Autodesk Inventor part; units mm, degrees
ref_plane "YZ Plane" through (0, 0, 0) normal (1, 0, 0) x (0, 1, 0)
ref_plane "XZ Plane" through (0, 0, 0) normal (0, 1, 0) x (-1, 0, 0)
ref_plane "XY Plane" through (0, 0, 0) normal (0, 0, 1) x (1, 0, 0)
sketch "Sketch1" plane through (0, 0, 0) normal (0, 1, 0) x (-1, 0, 0)
  line L0 (15.5575, -22.86) -> (15.5575, 27.94)
  line L1 (15.5575, 27.94) -> (-15.5575, 27.94)
  line L2 (-15.5575, 27.94) -> (-15.5575, -22.86)
  line L3 (-15.5575, -27.94) -> (15.5575, 27.94) construction
  line L4 (15.5575, -27.94) -> (-15.5575, 27.94) construction
  line L5 (20.6375, -27.94) -> (20.955, -27.94)
  line L6 (20.955, -27.94) -> (20.955, -78.74)
  line L7 (8.255, -91.44) -> (-8.255, -91.44)
  line L8 (-20.955, -78.74) -> (-20.955, -27.94)
  line L9 (-20.955, -27.94) -> (-20.6375, -27.94)
  arc A0 (15.5575, -22.86) -> (20.6375, -27.94) centre (20.6375, -22.86) ccw
  arc A1 (-20.6375, -27.94) -> (-15.5575, -22.86) centre (-20.6375, -22.86) ccw
  circle A2 centre (0, 7.3025) radius 9.525
  arc A3 (8.255, -91.44) -> (20.955, -78.74) centre (8.255, -78.74) ccw
  arc A4 (-20.955, -78.74) -> (-8.255, -91.44) centre (-8.255, -78.74) ccw
  circle A5 centre (0, -66.04) radius 7.366
  line L10 (0, 46.0525) -> (0, -103.086)
  circle A6 centre (7.62, 21.59) radius 2.3813
  circle A7 centre (-7.62, 21.59) radius 2.3813
  circle A8 centre (12.5412, -34.29) radius 2.3813
  circle A9 centre (-12.5412, -34.29) radius 2.3813
  point P0 (0, 0)
  point P1 (20.955, -91.44)
  point P2 (-20.955, -91.44)
  point P3 (0, 0)
  dimension "d0" = 5.08
  dimension "d1" = 31.115
  dimension "d2" = 41.91
  dimension "d3" = 63.5
  dimension "d4" = 119.38
  dimension "d5" = 19.05
  dimension "d6" = 20.6375
  dimension "d7" = 12.7
  dimension "d27" = 25.4
  dimension "d28" = 14.732
  dimension "d29" = 4.7625
  dimension "d30" = 15.24
  dimension "d31" = 6.35
  dimension "d32" = 25.0825
  dimension "d33" = 4.7625
  dimension "d34" = 57.15
extrude "Extrusion1" add sketch "Sketch1" along normal blind 12.7 contours A0 L5 L6 A3 L7 L10 A5 A2 L1 L0 | L10 A2 A5 L7 A4 L8 L9 A1 L2 L1
sketch "Sketch4" plane through (0, 0, 0) normal (0, -1, 0) x (1, 0, 0)
  circle A0 centre (0, -66.04) radius 7.366
  circle A1 centre (0, -66.04) radius 19.05
  point P0 (0, 0)
  dimension "d38" = 38.1
extrude "Extrusion3" cut sketch "Sketch4" against normal blind 2.54
chamfer "Chamfer1" distance 2.9464 angle 41 2 edges at (10.0013, 0, 21.59) (-5.2387, 0, 21.59) measured on face at (-0.3827, 0, -15.9577)
chamfer "Chamfer2" distance 2.9464 angle 41 2 edges at (-10.16, 12.7, -34.29) (14.9225, 12.7, -34.29) measured on face at (-0.3827, 12.7, -15.9577)
equation "\"d33\" = d29"
properties part number "Fixture_Airpot_Support"
Could you check a few things on this model? Use its own coordinates, in mm. A direction names the side the tool comes from. Round coordinates to 2 decimals unless told otherwise and drop trailing zeros. Write each loop counter-clockwise with the first axis right and the second up, starting at its lowest first coordinate (ties: lowest second). Pieces come first, ordered by that corner, then holes. Notation, with made-up numbers: (32.5, 57) - (52.5, 57) arc R31 ccw to (52.5, 91) - close; hole circle Ø10 at (30.25, 25). An arc over 180 degrees is marked (long way). Put each result on its own line as item: value. Start each with the question number.
(1) I need wall thicknesses on probe 1 along Z at (x, y) = (0, 0.75); probe 2 along Z at (x, y) = (6, 6.25); probe 3 along Z at (x, y) = (-3.5, 4). Which ranges of each line are inside material? Lowest first, please.
(2) Will these pins go through, and if not, where does the flat tip stop? pin 1 (4 mm diameter, centred on x = 13, y = 4, fed in from -Z); pin 2 (4 mm diameter, centred on y = 3.5, z = -4, fed in from +X); pin 3 (3 mm diameter, centred on y = 5.5, z = -12, fed in from -X).
(3) I want a section at B-B, the plane x = 0. Please give me the cut outline in (y, z).
(4) I want a section at C-C, the plane z = 21.59. Please give me the cut outline in (x, y), plus the area to 3 significant figures.
(5) Thinking about a two-plate mould opening in Z: for faces 4 (the cylindrical face through (-7.026, 7.549, -68.253)), 5 (the flat face through (-20.955, 6, -53)), 6 (the flat face through (0, 6, -91.44)), which applies, released by +Z, released by -Z, zero draft, split by the parting line, or undercut?
(6) I want a section at D-D, the plane y = 5.75. Give the number of separate pieces and of enclosed holes in the cut face, plus the area to 3 significant figures.
(7) For faces 1 (the flat face through (8, 2.54, -66)), 2 (the cylindrical face through (-17.333, 6.261, -87.621)), 3 (the flat face through (-15.558, 6, 2)), which set-ups out of +Z, -Z, +X, -X, +Y, -Y let a thin tool reach every point of the face, with its end or its side?
(8) I want a section at A-A, the plane z = -66.04. Please give me the cut outline in (x, y) (3 decimals).
Here are the results:
1. probe 1: z = -91.44 to -85.09, -46.99 to -2.22, 16.83 to 27.94
1. probe 2: z = -91.44 to -70.31, -61.77 to -0.1, 14.7 to 19.84, 23.34 to 27.94
1. probe 3: z = -91.44 to -72.52, -59.56 to -1.56, 16.16 to 27.94
2. pin 1: stops at z = -91.14
2. pin 2: stops at x = 15.56
2. pin 3: stops at x = -15.56
3. outline: (0, -91.44) - (12.7, -91.44) - (12.7, -73.41) - (2.54, -73.41) - (2.54, -85.09) - (0, -85.09) - close; (0, -46.99) - (2.54, -46.99) - (2.54, -58.67) - (12.7, -58.67) - (12.7, -2.22) - (0, -2.22) - close; (0, 16.83) - (12.7, 16.83) - (12.7, 27.94) - (0, 27.94) - close
4. outline: (-15.56, 0) - (-12.95, 0) - (-10, 2.56) - (-10, 12.7) - (-15.56, 12.7) - close; (-5.24, 2.56) - (-2.29, 0) - (2.29, 0) - (5.24, 2.56) - (5.24, 12.7) - (-5.24, 12.7) - close; (10, 2.56) - (12.95, 0) - (15.56, 0) - (15.56, 12.7) - (10, 12.7) - close
4. area: 259 mm^2
5. face 4: undercut
5. face 5: zero draft
5. face 6: released by -Z
6. separate pieces: 1
6. enclosed holes: 6
6. area: 3,820 mm^2
7. face 1: -Y
7. face 2: -Z, -X, +Y, -Y
7. face 3: +Z, -X, +Y, -Y
8. outline: (-20.955, 0) - (-19.05, 0) - (-19.05, 2.54) - (-7.366, 2.54) - (-7.366, 12.7) - (-20.955, 12.7) - close; (7.366, 2.54) - (19.05, 2.54) - (19.05, 0) - (20.955, 0) - (20.955, 12.7) - (7.366, 12.7) - close
